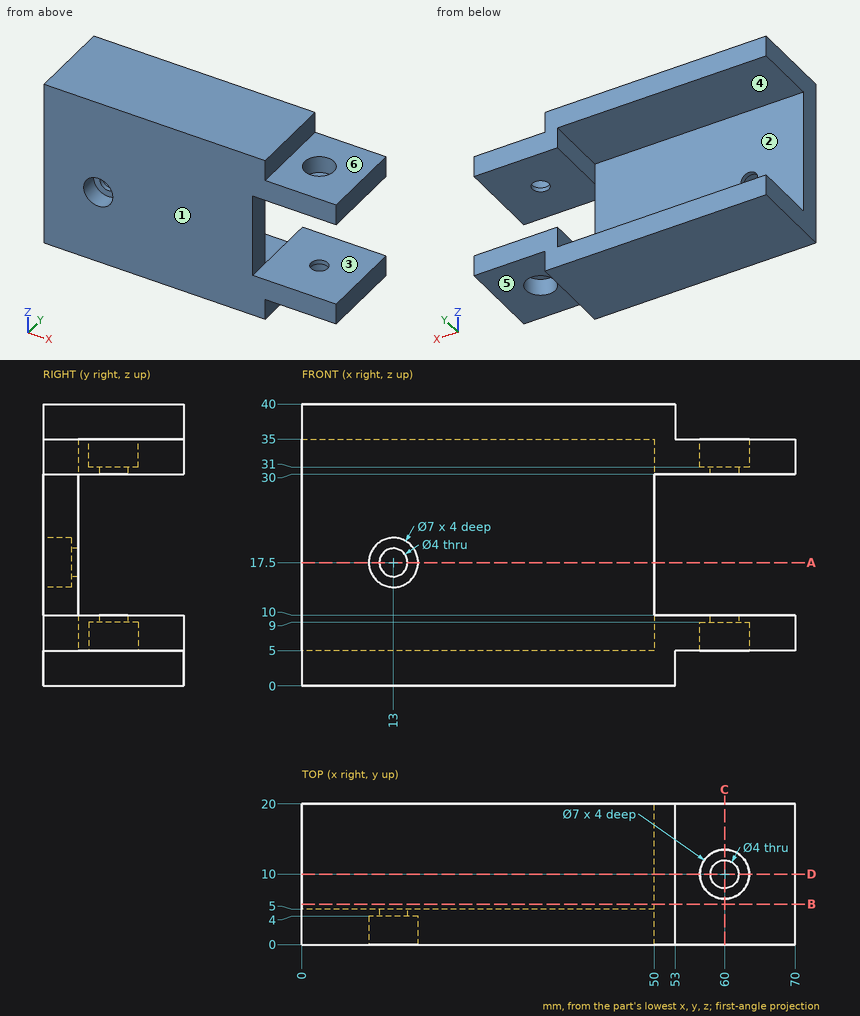
Design review of the part shown in the three views and the two pictorial views. Dimensions are in mm from the part's minimum x, y and z. A direction names the side the tool comes from. Round coordinates to 2 decimals unless told otherwise and drop trailing zeros. Order: outer loops, then holes, each group sorted by start corner. A loop starts at its lowest first (then second) coordinate and runs counter-clockwise, first axis right, second up. Notation, with made-up numbers: (89, 51) - (111, 51) arc R26 cw to (111, 68) - close; hole circle Ø8 at (-37.75, 85.25). An arc over 180 degrees is marked (long way). Answer in a Markdown table with one row per item.
(1) Machinability: for the marked faces 1, 2 and 3, which of the approach directions +Z, -Z, +X, -X, +Y, -Y give a long, thin tool a straight path to every point of the face, cutting with its end or side? Answer none if there is none.
Result set:
| item | result |
|---|---|
| face 1 | +Z, -Z, +X, -X, -Y |
| face 2 | -X, +Y |
| face 3 | +X, +Y, -Y |
(2) Clearance check with flat-ended pins moving along their axes: P1, Ø5, axis at y = 5.5, z = 18, coming from the -X side; P2, Ø6, axis at x = 58, y = 10, coming from the -Z side; P3, Ø5.5, axis at x = 60, y = 10, coming from the -Z side; P4, Ø12, axis at y = 13, z = 19.5, coming from the +X side. State where each tip first meets the part, or that it passes through.
Result set:
| item | result |
|---|---|
| P1 | stops at x = 0 |
| P2 | stops at z = 5 |
| P3 | stops at z = 9 |
| P4 | passes through |
(3) Take a section at C-C on x = 60. Write out the cut boundary in (y, z).
Result set:
| item | result |
|---|---|
| outline | (0, 5) - (6.5, 5) - (6.5, 9) - (8, 9) - (8, 10) - (0, 10) - close; (0, 30) - (8, 30) - (8, 31) - (6.5, 31) - (6.5, 35) - (0, 35) - close; (12, 9) - (13.5, 9) - (13.5, 5) - (20, 5) - (20, 10) - (12, 10) - close; (12, 30) - (20, 30) - (20, 35) - (13.5, 35) - (13.5, 31) - (12, 31) - close |
(4) For line 1 (Z direction, x = 66.5, y = 4.75); line 2 (Z direction, x = 38.5, y = 11.75); line 3 (Y direction, x = 16, z = 21), list the stretches that pass through material, from the lowest coordinate up. Write a range as from..to.
Result set:
| item | result |
|---|---|
| line 1 | z = 5..10, 30..35 |
| line 2 | z = 0..5, 35..40 |
| line 3 | y = 0..5 |
(5) Take a section at D-D on y = 10. Count the separate pieces of the cut face and the enclosed holes in it, plus the area to 3 significant figures.
Result set:
| item | result |
|---|---|
| separate pieces | 4 |
| enclosed holes | 0 |
| area | 666 mm2 |
(6) Mouldability with a two-part tool opening along Z and no side actions: class the marked faces 4, 5 and 6 as released by +Z, released by -Z, zero draft, split by the parting line, or undercut.
Result set:
| item | result |
|---|---|
| face 4 | undercut |
| face 5 | released by -Z |
| face 6 | released by +Z |
(7) Take a section at A-A on z = 17.5. Write out the cut boundary in (x, y), plus the area to 3 significant figures.
Result set:
| item | result |
|---|---|
| outline | (0, 0) - (9.5, 0) - (9.5, 4) - (11, 4) - (11, 5) - (0, 5) - close; (15, 4) - (16.5, 4) - (16.5, 0) - (50, 0) - (50, 5) - (15, 5) - close |
| area | 218 mm2 |
(8) Take a section at B-B on y = 5.75. Write out the cut boundary in (x, z), plus the area to 3 significant figures.
Result set:
| item | result |
|---|---|
| outline | (0, 0) - (53, 0) - (53, 5) - (70, 5) - (70, 10) - (50, 10) - (50, 5) - (0, 5) - close; (0, 35) - (50, 35) - (50, 30) - (70, 30) - (70, 35) - (53, 35) - (53, 40) - (0, 40) - close |
| area | 730 mm2 |
